from build123d import *

# Parameters (mm, degrees)
F0_R      = 1.05
F1_DEPTH  = 1.3
F3_W      = 2.2
F3_H      = 23
F4_DEPTH  = 0.7
F5_W      = 2.5
F5_H      = 1.5
F5_W_2    = 1.5
F5_H_2    = 2.5
F5_W_3    = 3
F5_W_4    = 2.2
F5_H_3    = 23
F6_DEPTH  = 0.9
F7_R      = 0.3
F8_R      = 0.3
F9_W      = 2
F9_H      = 1
F9_H_2    = 14
F10_DEPTH = 0.9
F3_W_2    = 3
F3_H_2    = 1.5
F3_W_3    = 1.5
F3_H_3    = 2.5
F11_DEPTH = 0.9


with BuildPart() as f1:
    # F0 (on Top) → F1 (new body)
    with BuildSketch(Plane.XY):
        Polygon((21.3, -14), (32, -14), (32, 14), (21.3, 14), (21.3, 11.5), (19.1, 11.5), (19.1, 14), (1.3, 14), (1.3, 11.5), (-0.9, 11.5), (-0.9, 14), (-32, 14), (-32, -14), (-0.9, -14), (-0.9, -11.5), (1.3, -11.5), (1.3, -14), (19.1, -14), (19.1, -11.5), (21.3, -11.5), align=None)
        with Locations((-24.5, -11)):
            Circle(F0_R, mode=Mode.SUBTRACT)
        Polygon((-10, 7), (-10, 5.1), (-8.5, 5.1), (-8.5, 7), (11.5, 7), (11.5, 5.1), (29.6, 5.1), (29.6, -5.1), (11.5, -5.1), (11.5, -7), (-8.5, -7), (-8.5, -5.1), (-10, -5.1), (-10, -7), (-30.5, -7), (-30.5, -5.1), (-30.5, 5.1), (-30.5, 7), align=None, mode=Mode.SUBTRACT)
        with Locations((-24.5, 11)):
            Circle(F0_R, mode=Mode.SUBTRACT)
    extrude(amount=F1_DEPTH)

    # F3 (on face) → F4 (join)
    with BuildSketch(Plane.XY.offset(1.3)):
        with Locations((30.9, 0)):
            Rectangle(F3_W, F3_H)
    extrude(amount=F4_DEPTH)

    # F5 (on face) → F6 (join)
    with BuildSketch(Plane(origin=(0, 0, 0), x_dir=(1, 0, 0), z_dir=(0, 0, -1))):
        with Locations((-10.65, 12.3576217964)):
            Rectangle(F5_W, F5_H)
        with Locations((-14.15, 9.75)):
            Rectangle(F5_W_2, F5_H_2)
        with Locations((-14.15, -9.75)):
            Rectangle(F5_W_2, F5_H_2)
        with Locations((-10.65, -12.3576217964)):
            Rectangle(F5_W, F5_H)
        with Locations((24.5, -12.15)):
            Rectangle(F5_W_3, F5_H)
        with Locations((30.9, 0)):
            Rectangle(F5_W_4, F5_H_3)
        with Locations((24.5, 12.15)):
            Rectangle(F5_W_3, F5_H)
    extrude(amount=F6_DEPTH)

    # F7
    f7_edges = [f1.edges().sort_by_distance(p)[0] for p in [
        (32, 0, -0.9),
    ]]
    fillet(f7_edges, radius=F7_R)

    # F8
    f8_edges = [f1.edges().sort_by_distance(p)[0] for p in [
        (32, 0, 2),
    ]]
    fillet(f8_edges, radius=F8_R)

    # F9 (on face) → F10 (join)
    with BuildSketch(Plane(origin=(0, 0, 0), x_dir=(1, 0, 0), z_dir=(0, 0, -1))):
        with Locations((-20.5, 7.5)):
            Rectangle(F9_W, F9_H)
        with Locations((-20.5, -7.5)):
            Rectangle(F9_W, F9_H)
        with Locations((-20.5, 0)):
            Rectangle(F9_W, F9_H_2)
    extrude(amount=F10_DEPTH)

    # F3 (on face) → F11 (join)
    with BuildSketch(Plane.XY.offset(1.3)):
        with Locations((-10.4, 12.15)):
            Rectangle(F3_W_2, F3_H_2)
        with Locations((-14.15, 9.75)):
            Rectangle(F3_W_3, F3_H_3)
        with Locations((-14.15, -9.75)):
            Rectangle(F3_W_3, F3_H_3)
        with Locations((-10.4, -12.15)):
            Rectangle(F3_W_2, F3_H_2)
        with Locations((24.5, -12.15)):
            Rectangle(F3_W_2, F3_H_2)
        with Locations((24.5, 12.15)):
            Rectangle(F3_W_2, F3_H_2)
    extrude(amount=F11_DEPTH)


solid = f1.part
Can you work these out from the model? Positions are in its coordinate system, mm. A direction names the side the tool comes from. Coordinates: 2 decimals unless noted, no trailing zeros. Write each loop counter-clockwise with the first axis right and the second up, starting at its lowest first coordinate (ties: lowest second). Pieces come first, ordered by that corner, then holes. Notation, with made-up numbers: (-3, 78.25) - (5, 78.25) arc R10 cw to (5, 96.25) - close; hole circle Ø5 at (82, 29). An arc over 180 degrees is marked (long way). Return JSON: item names as keys, results as strings. Group by question number.
Item 1: Please list where these lines run through material, in increasing order: probe 1 along Y at (x, z) = (-24.5, 0.8); probe 2 along Y at (x, z) = (-3.5, 1.2); probe 3 along Y at (x, z) = (27, 0.75).
Item 2: If we section it at D-D (x = 5.5): Write out the boundary of the cut face in (y, z), then the cut area to 3 significant figures.
Item 3: We'd pull the mould along X, two halves only. Please class faces 5 (the face through (-16, 14, 1)), 6 (the face through (21.3, 13, 1)): pulls with the +X half, pulls with the -X half, needs draft (parallel to the pull), parting line crosses it, or undercut.
Item 4: Which directions (+Z, -Z, +X, -X, +Y, -Y) give clear straight access to the entire face, cutting with the end or side of a thin tool? Please do faces 1 (the face through (-21, 0, 0)), 2 (the face through (11.5, -6, 1)), 3 (the face through (20, -11.5, 1)), 4 (the face through (31, 0, 2)).
Item 5: If we section it at B-B (y = 3.5): Write out the boundary of the cut face in (x, z).
Item 6: I'm going to push flat-ended pins straight in: pin 1 Ø0.7 at (y, z) = (-12, -0.5) entering from +X; pin 2 Ø8 at (x, y) = (4.5, 3.5) entering from -Z; pin 3 Ø10 at (x, y) = (-16, -3) entering from +Z; pin 4 Ø6 at (x, y) = (-0.5, -3.5) entering from -Z. Where does each tip first touch, or does it pass through?
Item 7: If we section it at A-A (x = 13): Write out the boundary of the cut face in (y, z).
Item 8: If we section it at C-C (x = -24.5): Write out the boundary of the cut face in (y, z), then the cut area to 3 significant figures.
Return value:
{
 "1": {"probe 1": "y = -14 to -12.05, -9.95 to -7, 7 to 9.95, 12.05 to 14", "probe 2": "y = -14 to -7, 7 to 14", "probe 3": "y = -14 to -5.1, 5.1 to 14"},
 "2": {"outline": "(-14, 0) - (-7, 0) - (-7, 1.3) - (-14, 1.3) - close; (7, 0) - (14, 0) - (14, 1.3) - (7, 1.3) - close", "area": "18.2 mm^2"},
 "3": {"face 5": "needs draft", "face 6": "undercut"},
 "4": {"face 1": "+Z", "face 2": "+Z, -Z", "face 3": "+Z, -Z, -Y", "face 4": "+Z, +X, +Y, -Y"},
 "5": {"outline": "(-32, 0) - (-30.5, 0) - (-30.5, 1.3) - (-32, 1.3) - close; (-21.5, -0.9) - (-19.5, -0.9) - (-19.5, 0) - (-21.5, 0) - close; (29.6, 0) - (29.8, 0) - (29.8, -0.9) - (31.7, -0.9) arc R0.3 ccw to (32, -0.6) - (32, 1.7) arc R0.3 ccw to (31.7, 2) - (29.8, 2) - (29.8, 1.3) - (29.6, 1.3) - close"},
 "6": {"pin 1": "stops at x = 26", "pin 2": "stops at z = 0", "pin 3": "stops at z = 1.3", "pin 4": "passes through"},
 "7": {"outline": "(-14, 0) - (-5.1, 0) - (-5.1, 1.3) - (-14, 1.3) - close; (5.1, 0) - (14, 0) - (14, 1.3) - (5.1, 1.3) - close"},
 "8": {"outline": "(-14, 0) - (-12.05, 0) - (-12.05, 1.3) - (-14, 1.3) - close; (-9.95, 0) - (-7, 0) - (-7, 1.3) - (-9.95, 1.3) - close; (7, 0) - (9.95, 0) - (9.95, 1.3) - (7, 1.3) - close; (12.05, 0) - (14, 0) - (14, 1.3) - (12.05, 1.3) - close", "area": "12.7 mm^2"}
}
